Here's how the part is built. I have some questions about the finished solid (model axes, mm). A direction names the side the tool comes from. Round coordinates to 2 decimals unless told otherwise and drop trailing zeros. Write each loop counter-clockwise with the first axis right and the second up, starting at its lowest first coordinate (ties: lowest second). Pieces come first, ordered by that corner, then holes. Notation, with made-up numbers: (-2.75, 45.25) - (55.25, 45.25) arc R15 ccw to (55.25, 65.25) - close; hole circle Ø3 at (64.25, 12). An arc over 180 degrees is marked (long way). Use one line per item in the form item = value. Start each with the question number.
1. Will these pins go through, and if not, where does the flat tip stop? pin 1 (1.2 mm diameter, centred on x = 5.5, z = -12, fed in from -Y); pin 2 (6.5 mm diameter, centred on x = 6.35, z = -12.7, fed in from +Y); pin 3 (1.9 mm diameter, centred on x = 7, y = 11.5, fed in from +Z).
2. I want a section at C-C, the plane y = 3.75. List the corners of the cut face in (x, z) for me.
3. We'd pull the mould along X, two halves only. Please class faces 6 (the flat face through (6, 7.3, -64)), 7 (the flat face through (6, 7, -13)), 8 (the flat face through (0, 2, -38)): +X half, -X half, draft (parallel to the pull), parting line (faces both ways), or undercut.
4. Which directions (+Z, -Z, +X, -X, +Y, -Y) give clear straight access to the entire face, cutting with the end or side of a thin tool? Please do faces 1 (the cylindrical face through (6.261, 26.347, -38.379)), 2 (the flat face through (6, 7, -63)), 3 (the cylindrical face through (3.13, 21.08, -46.21)), 4 (the flat face through (6, 7.3, -13)), 5 (the flat face through (6, 10, -50.8)).
5. I want a section at D-D, the plane y = 8.5. List the corners of the cut face in (x, z) for me.
6. If I drill on line 1 along Y through (x, z) = (2.5, -38.1); line 2 along Y through (x, z) = (7.75, -19); line 3 along Y through (x, z) = (7, -13), over which ranges is the centre line in solid material (lowest first)?
7. I want a section at A-A, the plane z = -38.1. List the corners of the cut face in (x, y) for me (3 decimals).
8. I want a section at B-B, the plane x = 9.75. List the corners of the cut face in (y, z) for me (3 decimals), plus the area to 3 significant figures.
```python
from build123d import *

# Parameters (mm, degrees)
BOSS_EXTRUDE1_DEPTH = 12.7
SKETCH2_R           = 7.62500004
CUT_EXTRUDE1_DEPTH  = 82.621397317
SKETCH3_R           = 2
CUT_EXTRUDE2_DEPTH  = 7
SKETCH4_R           = 11
CUT_EXTRUDE3_DEPTH  = 6.35


with BuildPart() as part:
    # Sketch1 → Boss-Extrude1 (new body)
    with BuildSketch(Plane(origin=(0, 0, 0), x_dir=(0, 0, -1), z_dir=(1, 0, 0))):
        with BuildLine():
            Line((0, 0), (76.2, 0))
            Line((76.2, 0), (76.2, 7.3))
            Line((76.2, 7.3), (50.8, 7.3))
            Line((50.8, 7.3), (50.8, 13.65))
            ThreePointArc((50.8, 13.65), (38.1, 26.35), (25.4, 13.65))
            Line((25.4, 13.65), (25.4, 7.3))
            Line((25.4, 7.3), (0, 7.3))
            Line((0, 7.3), (0, 0))
        make_face()
    extrude(amount=BOSS_EXTRUDE1_DEPTH)

    # Sketch2 → Cut-Extrude1 (cut, through all)
    with BuildSketch(Plane(origin=(12.7, 0, 0), x_dir=(0, 0, -1), z_dir=(1, 0, 0))):
        with Locations((38.1, 13.65)):
            Circle(SKETCH2_R)
    extrude(amount=-CUT_EXTRUDE1_DEPTH, mode=Mode.SUBTRACT)

    # Sketch3 → Cut-Extrude2 (cut)
    with BuildSketch(Plane.XZ):
        with Locations(Location((6.35, -12.7, 0), (0, 0, 270))):
            Circle(SKETCH3_R)
        with Locations(Location((6.35, -63.5, 0), (0, 0, 270))):
            Circle(SKETCH3_R)
    extrude(amount=-CUT_EXTRUDE2_DEPTH, mode=Mode.SUBTRACT)

    # Sketch4 → Cut-Extrude3 (cut)
    with BuildSketch(Plane.ZY):
        with Locations((-38.1, 13.65)):
            Circle(SKETCH4_R)
    extrude(amount=-CUT_EXTRUDE3_DEPTH, mode=Mode.SUBTRACT)


solid = part.part
```
Model answer:
q1.pin_1 = 7
q1.pin_2 = 7.3
q1.pin_3 = -25.4
q2.outline = (0, -76.2) - (12.7, -76.2) - (12.7, 0) - (0, 0) - (0, -33.31) - (6.35, -33.31) - (6.35, -42.89) - (0, -42.89) - close; hole circle Ø4 at (6.35, -63.5); hole circle Ø4 at (6.35, -12.7)
q3.face_6 = draft
q3.face_7 = undercut
q3.face_8 = -X half
q4.face_1 = +X, -X, +Y
q4.face_2 = -Y
q4.face_3 = -X
q4.face_4 = +Z, +X, -X, +Y
q4.face_5 = -Z, +X, -X, +Y
q5.outline = (0, -50.8) - (12.7, -50.8) - (12.7, -43.72) - (6.35, -43.72) - (6.35, -47.82) - (0, -47.82) - close; (0, -28.38) - (6.35, -28.38) - (6.35, -32.48) - (12.7, -32.48) - (12.7, -25.4) - (0, -25.4) - close
q6.line_1 = 0 to 2.65, 24.65 to 26.35
q6.line_2 = 0 to 7.3
q6.line_3 = 7 to 7.3
q7.outline = (0, 0) - (12.7, 0) - (12.7, 6.025) - (6.35, 6.025) - (6.35, 2.65) - (0, 2.65) - close; (0, 24.65) - (6.35, 24.65) - (6.35, 21.275) - (12.7, 21.275) - (12.7, 26.35) - (0, 26.35) - close
q8.outline = (0, -76.2) - (7.3, -76.2) - (7.3, -50.8) - (13.65, -50.8) arc R12.7 ccw to (13.65, -25.4) - (7.3, -25.4) - (7.3, 0) - (0, 0) - close; hole circle Ø15.25 at (13.65, -38.1)
q8.area = 788 mm2
